```python
from build123d import *

# Parameters (mm, degrees)
SALIENTE_EXTRUIR1_DEPTH = 35
CROQUIS2_W              = 3
CROQUIS2_H              = 24
CORTAR_EXTRUIR1_DEPTH   = 22


with BuildPart() as part:
    # Croquis1 → Saliente-Extruir1 (new body)
    with BuildSketch(Plane(origin=(0, 0, 0), x_dir=(1, 0, 0), z_dir=(0, 1, 0))):
        with BuildLine():
            Line((-23, 0), (-70, 0))
            Line((-70, 0), (-70, -70))
            Line((-70, -70), (-23, -70))
            ThreePointArc((-23, -70), (-6.736544033, -63.263455967), (0, -47))
            Line((0, -47), (0, -23))
            ThreePointArc((0, -23), (-6.736544033, -6.736544033), (-23, 0))
        make_face()
    extrude(amount=SALIENTE_EXTRUIR1_DEPTH)

    # Croquis2 → Cortar-Extruir1 (cut)
    with BuildSketch(Plane(origin=(0, 0, 0), x_dir=(-1, 0, 0), z_dir=(0, 0, -1))):
        with Locations((66.5, 17.5)):
            Rectangle(CROQUIS2_W, CROQUIS2_H)
    extrude(amount=-CORTAR_EXTRUIR1_DEPTH, mode=Mode.SUBTRACT)


solid = part.part
```
The listing builds one solid part. Answer for the finished solid, in the listing's coordinates (mm). A direction names the side the tool comes from. Round coordinates to 2 decimals unless told otherwise and drop trailing zeros. Write each loop counter-clockwise with the first axis right and the second up, starting at its lowest first coordinate (ties: lowest second). Pieces come first, ordered by that corner, then holes. Notation, with made-up numbers: (-28, 57) -> (-2, 57) arc R27 ccw to (-2, 74) -> close; hole circle Ø1 at (-17.5, 65.5). An arc over 180 degrees is marked (long way). Answer as a JSON object with one key per item and string values. Group by question number.
Q1. Determine the mould class of faces 1 (the face through (-65, 17, 11)), 2 (the face through (-47, 17, 70)), 3 (the face through (-35, 0, 35)) for opening direction Y: pulls with the +Y half, pulls with the -Y half, needs draft (parallel to the pull), parting line crosses it, or undercut.
Q2. Section B-B (z = 8) is taken. Write down the section's boundary in (x, y).
Q3. Each of these flat-tipped pins is pushed along its axis until it touches: pin 1 Ø2 at (y, z) = (4.5, 62) entering from +X; pin 2 Ø3 at (y, z) = (26, 13) entering from +X; pin 3 Ø2.5 at (x, y) = (-66.5, 19) entering from -Z. Where does it stop, or does it pass through?
Q4. Section A-A (y = 27) is taken. Write down the section's boundary in (x, z), plus the area to 3 significant figures.
Q5. Straight lines are drawn through the part: line 1 along X through (y, z) = (15, 15); line 2 along Z through (x, y) = (-66.5, 10); line 3 along X through (y, z) = (21.5, 15.5). For each, find the intervals that lie inside material, in ascending order.
Q6. Section C-C (z = 19) is taken. Write down the section's boundary in (x, y), plus the area to 3 significant figures.
Q7. Which of the six approach directions +Z, -Z, +X, -X, +Y, -Y give full straight-line access (tool end or side, diameter ignored) to faces 4 (the face through (-68, 17, 11)), 5 (the face through (-6.559, 17.255, 6.916))?
Q8. Section D-D (x = -12) is taken. Write down the section's boundary in (y, z).
Check values:
{
 "1": {"face 1": "undercut", "face 2": "needs draft", "face 3": "pulls with the -Y half"},
 "2": {"outline": "(-70, 0) -> (-5.56, 0) -> (-5.56, 35) -> (-70, 35) -> close; hole (-68, 5.5) -> (-65, 5.5) -> (-65, 29.5) -> (-68, 29.5) -> close"},
 "3": {"pin 1": "x = -4.75", "pin 2": "x = -1.63", "pin 3": "z = 22"},
 "4": {"outline": "(-70, 0) -> (-68, 0) -> (-68, 22) -> (-65, 22) -> (-65, 0) -> (-23, 0) arc R23 ccw to (0, 23) -> (0, 47) arc R23 ccw to (-23, 70) -> (-70, 70) -> close", "area": "4,610 mm^2"},
 "5": {"line 1": "-70 to -68, -65 to -1.44", "line 2": "22 to 70", "line 3": "-70 to -68, -65 to -1.26"},
 "6": {"outline": "(-70, 0) -> (-0.35, 0) -> (-0.35, 35) -> (-70, 35) -> close; hole (-68, 5.5) -> (-65, 5.5) -> (-65, 29.5) -> (-68, 29.5) -> close", "area": "2,370 mm^2"},
 "7": {"face 4": "-Z", "face 5": "-Z, +X, +Y, -Y"},
 "8": {"outline": "(0, 2.8) -> (35, 2.8) -> (35, 67.2) -> (0, 67.2) -> close"}
}
